Autodesk Inventor part; units mm, degrees
ref_plane "YZ Plane" through (0, 0, 0) normal (1, 0, 0) x (0, 1, 0)
ref_plane "XZ Plane" through (0, 0, 0) normal (0, 1, 0) x (-1, 0, 0)
ref_plane "XY Plane" through (0, 0, 0) normal (0, 0, 1) x (1, 0, 0)
sketch "Sketch1" plane through (0, 0, 0) normal (0, 1, 0) x (-1, 0, 0)
  circle A0 centre (0, 0) radius 20
  dimension "d0" = 40
extrude "Extrusion1" add sketch "Sketch1" along normal blind 2.6
sketch "Sketch2" plane through (0, 2.6, 0) normal (0, 1, 0) x (1, 0, 0)
  line L0 (-10, -10) -> (10, -10)
  line L1 (10, -10) -> (10, 10)
  line L2 (10, 10) -> (-10, 10)
  line L3 (-10, 10) -> (-10, -10)
  line L4 (-10, -10) -> (10, 10) construction
  line L5 (10, -10) -> (-10, 10) construction
  point P0 (0, 0)
  dimension "d3" = 20
  dimension "d4" = 20
extrude "Extrusion2" cut sketch "Sketch2" against normal blind 0.6
sketch "Sketch3" plane through (0, 2, 0) normal (0, 1, 0) x (1, 0, 0)
  line L0 (-6.2058, 8.5439) -> (6.2509, 8.5439) construction
  line L1 (6.2509, 8.5439) -> (6.2509, -8.4059) construction
  line L2 (6.2509, -8.4059) -> (-6.2058, -8.4059) construction
  line L3 (-6.2058, -8.4059) -> (-6.2058, 8.5439) construction
  line L4 (5.242, -8.4059) -> (-4.9952, -8.4059)
  line L5 (-4.9952, -8.4059) -> (-4.9952, -6.0518)
  spline S0 degree 2 poles (-4.9952, -6.0518) (-3.8921, -5.0159) (-1.9281, -3.0923) (-0.9864, -2.0565) knots 0 0 0 1 2 2 2
  spline S1 degree 2 poles (-0.9864, -2.0565) (0.9104, 0.0286) (2.2959, 2.5307) (2.2959, 3.8625) knots 0 0 0 1 2 2 2
  spline S2 degree 2 poles (2.2959, 3.8625) (2.2959, 4.562) (1.8655, 5.6113) (1.4754, 5.9476) knots 0 0 0 1 2 2 2
  spline S3 degree 2 poles (1.4754, 5.9476) (1.0852, 6.2839) (0.0629, 6.6202) (-0.5559, 6.6202) knots 0 0 0 1 2 2 2
  spline S4 degree 2 poles (-0.5559, 6.6202) (-1.1478, 6.6202) (-2.3585, 6.3243) (-2.9101, 6.0956) knots 0 0 0 1 2 2 2
  spline S5 degree 2 poles (-2.9101, 6.0956) (-3.3809, 5.9072) (-4.2553, 5.3691) (-4.5243, 5.1808) knots 0 0 0 1 2 2 2
  line L6 (-4.5243, 5.1808) -> (-4.6454, 5.1808)
  line L7 (-4.6454, 5.1808) -> (-4.6454, 7.5484)
  spline S6 degree 2 poles (-4.6454, 7.5484) (-3.9593, 7.8847) (-1.4976, 8.5439) (-0.3945, 8.5439) knots 0 0 0 1 2 2 2
  spline S7 degree 2 poles (-0.3945, 8.5439) (1.9327, 8.5439) (4.5559, 6.0821) (4.5559, 3.9836) knots 0 0 0 1 2 2 2
  spline S8 degree 2 poles (4.5559, 3.9836) (4.5559, 3.0016) (4.0985, 1.3604) (3.695, 0.6609) knots 0 0 0 1 2 2 2
  spline S9 degree 2 poles (3.695, 0.6609) (3.2914, -0.0655) (2.1211, -1.4915) (1.4754, -2.1775) knots 0 0 0 1 2 2 2
  spline S10 degree 2 poles (1.4754, -2.1775) (0.4261, -3.321) (-2.1433, -5.7693) (-2.9101, -6.4822) knots 0 0 0 1 2 2 2
  line L8 (-2.9101, -6.4822) -> (5.242, -6.4822)
  line L9 (5.242, -6.4822) -> (5.242, -8.4059)
  point P0 (0, 0)
extrude "Extrusion3" add sketch "Sketch3" along normal blind 0.6
properties part number "TopMarker2"
The model under review builds one solid part; all positions refer to its coordinate system, in mm. Round coordinates to 2 decimals unless told otherwise and drop trailing zeros. Loops run counter-clockwise (first coordinate to the right, second up) from the corner with the lowest first, then second, coordinate; pieces in that order, holes last.
Item 1: Take a section at D-D (x = 13.5). Write out the cut boundary in (y, z).
Determined:
outline: (0, -14.76) - (2.6, -14.76) - (2.6, 14.76) - (0, 14.76) - close
Item 2: Clearance check with flat-ended pins moving along their axes: pin 1 Ø0.7 at (x, y) = (-1.5, 2) entering from +Z; pin 2 Ø1 at (y, z) = (1.5, -8) entering from -X; pin 3 Ø0.7 at (y, z) = (2.5, -6.5) entering from -X. State where each tip first meets the part, or that it passes through.
Determined:
pin 1: stops at z = 19.97
pin 2: stops at x = -18.54
pin 3: stops at x = -19.03
Item 3: For line 1 (Z direction, x = 1.5, y = 2.3); line 2 (Z direction, x = -2, y = 2.4); line 3 (X direction, y = 2.4, z = 7.5), list the stretches that pass through material, from the lowest coordinate up.
Determined:
line 1: z = -19.94 to -10, -8.29 to -5.93, -1.1 to 2.15, 6.48 to 8.41, 10 to 19.94
line 2: z = -19.9 to -10, -8.38 to -6.41, 3.14 to 5.63, 6.48 to 8.41, 10 to 19.9
line 3: x = -18.54 to -10, -5 to 5.24, 10 to 18.54
Item 4: Take a section at A-A (x = -5.5). Write out the cut boundary in (y, z), then the cut area to 3 significant figures.
Determined:
outline: (0, -19.23) - (2.6, -19.23) - (2.6, -10) - (2, -10) - (2, 10) - (2.6, 10) - (2.6, 19.23) - (0, 19.23) - close
area: 88.0 mm2
Item 5: Take a section at C-C (y = 1). Write out the cut boundary in (x, z).
Determined:
outline: circle Ø40 at (0, 0)
Item 6: Take a section at B-B (z = -9). Write out the cut boundary in (x, y), then the cut area to 3 significant figures.
Determined:
outline: (-17.86, 0) - (17.86, 0) - (17.86, 2.6) - (10, 2.6) - (10, 2) - (-10, 2) - (-10, 2.6) - (-17.86, 2.6) - close
area: 80.9 mm2
Item 7: Mouldability with a two-part tool opening along X and no side actions: class faces 1 (the face through (0, 2, 0)), 2 (the face through (4.336, 1.282, 19.524)), 3 (the face through (0, 0, 0)) as released by +X, released by -X, zero draft, split by the parting line, or undercut.
Determined:
face 1: undercut
face 2: split by the parting line
face 3: zero draft
